Input: part model. Units: mm. Frame: model coordinates. Round coordinates to 2 decimals unless told otherwise and drop trailing zeros. Order: outer loops, then holes, each group sorted by start corner. A loop starts at its lowest first (then second) coordinate and runs counter-clockwise, first axis right, second up. Notation, with made-up numbers: (58.25, 41) -> (72.25, 41) arc R16 cw to (72.25, 46) -> close; hole circle Ø10 at (-12.5, -37). An arc over 180 degrees is marked (long way). Answer as CSV lines item,"result". Start each with the question number.
1) First-contact query: P1, Ø8, axis at x = -18, y = 0, coming from the -Z side; P2, Ø1.6, axis at x = 6.72, y = 6.72, coming from the -Z side; P3, Ø1.5, axis at x = 19.5, z = 1, coming from the +Y side; P4, Ø1.5, axis at y = -7.5, z = 0.5, coming from the -X side. Flat tips, straight axial feed; report the tip coordinate or a pass-through.
2) Line query: L1, parallel to Y at x = 0, z = 1.15; L2, parallel to X at y = -0.5, z = 1.15; L3, parallel to Y at x = 7, z = 0.6. Output: solid intervals per line, ascending.
3) Mould query, pull axis X, two halves, no side actions, for faces 1 (the face through (0, -6, 2.5)), 2 (the face through (-6.18, 7.56, 1.23)), 3 (the face through (25.865, -10.724, 1.268)). Classes: +X half, -X half, draft (parallel to the pull), parting line (faces both ways), or undercut.
4) Section query A-A, the plane y = 0. Output: boundary loops of the cut face in (x, z).
5) Section query C-C, the plane x = 25.2. Output: boundary loops of the cut face in (y, z), and give its area (3 significant figures).
6) Section query B-B, the plane z = 1.1. State how many separate pieces and enclosed holes the cut face has, and give its area (3 significant figures).
```python
from build123d import *

# Parameters (mm, degrees)
CROQUIS1_W              = 65
CROQUIS1_H              = 65
CROQUIS1_R              = 5.5
CROQUIS1_R_2            = 1
SALIENTE_EXTRUIR1_DEPTH = 2.5
REDONDEO1_R             = 15
CROQUIS5_R              = 47.665857464
CROQUIS5_R_2            = 28
CORTAR_EXTRUIR3_DEPTH   = 2.5
CROQUIS7_R              = 1
CORTAR_EXTRUIR4_DEPTH   = 2.5


with BuildPart() as part:
    # Croquis1 → Saliente-Extruir1 (new body)
    with BuildSketch(Plane.XY):
        Rectangle(CROQUIS1_W, CROQUIS1_H)
        Circle(CROQUIS1_R, mode=Mode.SUBTRACT)
        with Locations((-6.717514421, 6.717514421)):
            Circle(CROQUIS1_R_2, mode=Mode.SUBTRACT)
        with Locations((6.717514421, 6.717514421)):
            Circle(CROQUIS1_R_2, mode=Mode.SUBTRACT)
        with Locations((6.717514421, -6.717514421)):
            Circle(CROQUIS1_R_2, mode=Mode.SUBTRACT)
        with Locations((-6.717514421, -6.717514421)):
            Circle(CROQUIS1_R_2, mode=Mode.SUBTRACT)
    extrude(amount=SALIENTE_EXTRUIR1_DEPTH)

    # Redondeo1
    redondeo1_edges = [part.edges().sort_by_distance(p)[0] for p in [
        (32.5, -32.5, 1.25),
        (-32.5, -32.5, 1.25),
        (-32.5, 32.5, 1.25),
        (32.5, 32.5, 1.25),
    ]]
    fillet(redondeo1_edges, radius=REDONDEO1_R)

    # Croquis5 → Cortar-Extruir3 (cut)
    with BuildSketch(Plane.XY.offset(2.5)):
        Circle(CROQUIS5_R)
        Circle(CROQUIS5_R_2, mode=Mode.SUBTRACT)
    extrude(amount=-CORTAR_EXTRUIR3_DEPTH, mode=Mode.SUBTRACT)

    # Croquis7 → Cortar-Extruir4 (cut)
    with BuildSketch(Plane.XY.offset(2.5)):
        with Locations((0, 25.2)):
            Circle(CROQUIS7_R)
        with Locations((25.2, 0)):
            Circle(CROQUIS7_R)
        with Locations((0, -25.2)):
            Circle(CROQUIS7_R)
        with Locations((-25.2, 0)):
            Circle(CROQUIS7_R)
    extrude(amount=-CORTAR_EXTRUIR4_DEPTH, mode=Mode.SUBTRACT)


solid = part.part
```
Findings:
1,P1,"stops at z = 0"
1,P2,"passes through"
1,P3,"stops at y = 20.8"
1,P4,"stops at x = -27.17"
2,L1,"y = -28 to -26.2, -24.2 to -5.5, 5.5 to 24.2, 26.2 to 28"
2,L2,"x = -28 to -26.07, -24.33 to -5.48, 5.48 to 24.33, 26.07 to 28"
2,L3,"y = -27.11 to -7.68, -5.76 to 5.76, 7.68 to 27.11"
3,face 1,"draft"
3,face 2,"undercut"
3,face 3,"parting line"
4,outline,"(-28, 0) -> (-26.2, 0) -> (-26.2, 2.5) -> (-28, 2.5) -> close; (-24.2, 0) -> (-5.5, 0) -> (-5.5, 2.5) -> (-24.2, 2.5) -> close; (5.5, 0) -> (24.2, 0) -> (24.2, 2.5) -> (5.5, 2.5) -> close; (26.2, 0) -> (28, 0) -> (28, 2.5) -> (26.2, 2.5) -> close"
5,outline,"(-12.2, 0) -> (-1, 0) -> (-1, 2.5) -> (-12.2, 2.5) -> close; (1, 0) -> (12.2, 0) -> (12.2, 2.5) -> (1, 2.5) -> close"
5,area,"56.0 mm^2"
6,separate pieces,"1"
6,enclosed holes,"9"
6,area,"2,340 mm^2"
